Verification items for the finished model (mm, model axes). Coordinates: 2 decimals unless noted, no trailing zeros. Write each loop counter-clockwise with the first axis right and the second up, starting at its lowest first coordinate (ties: lowest second). Pieces come first, ordered by that corner, then holes. Notation, with made-up numbers: M -36.75,65.25 L 1.25,65.25 A28 ccw 1.25,92.25 Z; hole C 1.5,51.5 d5. An arc over 180 degrees is marked long. One line per item, written item: value.
```python
from build123d import *

# Parameters (mm, degrees)
SKETCH_1_W          = 44.5
SKETCH_1_H          = 30
EXTRUDE_1_DEPTH     = 3
SKETCH_2_R          = 1.6
SKETCH_2_R_2        = 2.1
CUT_EXTRUDE_1_DEPTH = 3
FILLET_1_R          = 5


with BuildPart() as part:
    # ｽｹｯﾁ1 → ﾎﾞｽ - 押し出し1 (new body)
    with BuildSketch(Plane(origin=(0, 0, 0), x_dir=(1, 0, 0), z_dir=(0, 1, 0))):
        with Locations((22.25, 15)):
            Rectangle(SKETCH_1_W, SKETCH_1_H)
    extrude(amount=EXTRUDE_1_DEPTH)

    # ｽｹｯﾁ2 → ｶｯﾄ - 押し出し1 (cut)
    with BuildSketch(Plane(origin=(0, 3, 0), x_dir=(1, 0, 0), z_dir=(0, 1, 0))):
        with Locations((3.75, 22.5)):
            Circle(SKETCH_2_R)
        with Locations((40.75, 22.5)):
            Circle(SKETCH_2_R)
        with Locations((3.75, 7.5)):
            Circle(SKETCH_2_R_2)
        with Locations((40.75, 7.5)):
            Circle(SKETCH_2_R_2)
    extrude(amount=-CUT_EXTRUDE_1_DEPTH, mode=Mode.SUBTRACT)

    # ﾌｨﾚｯﾄ1
    fillet_1_edges = [part.edges().sort_by_distance(p)[0] for p in [
        (0, 1.5, -30),
        (44.5, 1.5, -30),
        (44.5, 1.5, 0),
        (0, 1.5, 0),
    ]]
    fillet(fillet_1_edges, radius=FILLET_1_R)


solid = part.part
```
Item 1: Cross-section at B-B, the plane y = 1.85. Enter the section's corners in (x, z), and give its area (3 significant figures).
The answers:
outline: M 0,-25 A5 ccw 5,-30 L 39.5,-30 A5 ccw 44.5,-25 L 44.5,-5 A5 ccw 39.5,0 L 5,0 A5 ccw 0,-5 Z; hole C 3.75,-7.5 d4.2; hole C 3.75,-22.5 d3.2; hole C 40.75,-7.5 d4.2; hole C 40.75,-22.5 d3.2
area: 1,270 mm²
Item 2: Draft check along X on faces 1 (the face through (3.542, 1.521, -24.086)), 2 (the face through (1, 2, -28)), 3 (the face through (22, 3, -15)). Enter one of: released by +X, released by -X, zero draft, split by the parting line, or undercut.
The answers:
face 1: undercut
face 2: released by -X
face 3: zero draft
Item 3: Scan lines: line 1 (X direction, y = 1.7, z = -22.5); line 2 (X direction, y = 0.4, z = -5.75); line 3 (Z direction, x = 40.75, y = 2). Record each from-to range of solid material in increasing order.
The answers:
line 1: x = 0 to 2.15, 5.35 to 39.15, 42.35 to 44.5
line 2: x = 0 to 2.59, 4.91 to 39.59, 41.91 to 44.5
line 3: z = -29.84 to -24.1, -20.9 to -9.6, -5.4 to -0.16
Item 4: Cross-section at A-A, the plane z = -22.5. Enter the section's corners in (x, y).
The answers:
outline: M 0,0 L 2.15,0 L 2.15,3 L 0,3 Z; M 5.35,0 L 39.15,0 L 39.15,3 L 5.35,3 Z; M 42.35,0 L 44.5,0 L 44.5,3 L 42.35,3 Z
Item 5: Cross-section at C-C, the plane x = 3. Enter the section's corners in (y, z).
The answers:
outline: M 0,-29.58 L 3,-29.58 L 3,-23.91 L 0,-23.91 Z; M 0,-21.09 L 3,-21.09 L 3,-9.46 L 0,-9.46 Z; M 0,-5.54 L 3,-5.54 L 3,-0.42 L 0,-0.42 Z
